```python
from build123d import *

# Parameters (mm, degrees)
EXTRUDE_1_DEPTH        = 110
FILLET_1_R             = 0.2
SKETCH_2_R             = 5.5
CUT_EXTRUDE_1_DEPTH    = 8
SKETCH_3_R             = 3.5
CUT_EXTRUDE_2_DEPTH    = 124.081273962
HOLE_WIZARD_M4_1_D     = 3.3
HOLE_WIZARD_M4_1_DEPTH = 16.5
HOLE_WIZARD_M4_1_TIP   = 0.991420021


with BuildPart() as part:
    # 스케치1 → 보스-돌출1 (new body)
    with BuildSketch(Plane(origin=(0, 0, 0), x_dir=(1, 0, 0), z_dir=(0, 1, 0))):
        Polygon((0, -43), (0, 0), (45, 0), (45, -40), (3, -40), (3, -43), align=None)
    extrude(amount=EXTRUDE_1_DEPTH)

    # 필렛1
    fillet_1_edges = [part.edges().sort_by_distance(p)[0] for p in [
        (3, 55, 40),
    ]]
    fillet(fillet_1_edges, radius=FILLET_1_R)

    # 스케치2 → 컷-돌출1 (cut)
    with BuildSketch(Plane.XY.offset(40)):
        with Locations((12.5, 75)):
            Circle(SKETCH_2_R)
        with Locations((35.5, 75)):
            Circle(SKETCH_2_R)
        with Locations((12.5, 35)):
            Circle(SKETCH_2_R)
        with Locations((35.5, 35)):
            Circle(SKETCH_2_R)
    extrude(amount=-CUT_EXTRUDE_1_DEPTH, mode=Mode.SUBTRACT)

    # 스케치3 → 컷-돌출2 (cut, through all)
    with BuildSketch(Plane.XY.offset(32)):
        with Locations((12.5, 75)):
            Circle(SKETCH_3_R)
        with Locations((35.5, 75)):
            Circle(SKETCH_3_R)
        with Locations((35.5, 35)):
            Circle(SKETCH_3_R)
        with Locations((12.5, 35)):
            Circle(SKETCH_3_R)
    extrude(amount=-CUT_EXTRUDE_2_DEPTH, mode=Mode.SUBTRACT)

    # M4 나사 구멍1
    with Locations(Plane.XY.offset(40)):
        with Locations((12.5, 95), (12.5, 15), (12.5, 55), (35.5, 55), (35.5, 95), (35.5, 15)):
            Hole(HOLE_WIZARD_M4_1_D / 2, depth=HOLE_WIZARD_M4_1_DEPTH)
            with Locations((0, 0, -(HOLE_WIZARD_M4_1_DEPTH + HOLE_WIZARD_M4_1_TIP / 2))):  # 118° drill point
                Cone(0, HOLE_WIZARD_M4_1_D / 2, HOLE_WIZARD_M4_1_TIP, mode=Mode.SUBTRACT)


solid = part.part
```
Verification items for the finished model (mm, model axes). A direction names the side the tool comes from. Give positions to 0.01 mm unless a question says otherwise; leave off trailing zeros. Order: outer loops, then holes, each group sorted by start corner. A loop starts at its lowest first (then second) coordinate and runs counter-clockwise, first axis right, second up. Notation, with made-up numbers: M -9.75,75.25 L 1.25,75.25 A21 ccw 1.25,82.25 Z; hole C 78.5,60 d4. An arc over 180 degrees is marked long. Return JSON: item names as keys, results as strings. Group by question number.
1) Scan lines: line 1 (Y direction, x = 35.5, z = 35.5); line 2 (Y direction, x = 12.5, z = 31.25); line 3 (X direction, y = 55, z = 34). Record each from-to range of solid material in increasing order.
2) Access from +Z, -Z, +X, -X, +Y, -Y to the whole of each face (thin tool, end or side, straight path). Record for faces 1 (the face through (34.741, 71.583, 16.224)), 2 (the face through (35, 31, 32)), 3 (the face through (24, 54, 40)).
3) Section check D-D on z = 33.5. Give the number of separate pieces and of enclosed holes in the cut face, and give its area (3 significant figures).
4) Section check B-B on z = 21. Record the cut outline in (x, y), and give its area (3 significant figures).
5) Mould release check, pull along X, two halves, no side actions. Record for faces 4 (the face through (35.9, 93.4, 31.6)), 5 (the face through (0, 54, 22)), 6 (the face through (2, 54, 43)): pulls with the +X half, pulls with the -X half, needs draft (parallel to the pull), parting line crosses it, or undercut.
6) Go/stop test with flat-tipped pins: pin 1 Ø12 at (x, y) = (34.5, 37) entering from +Z; pin 2 Ø2.5 at (x, y) = (35.5, 15) entering from +Z; pin 3 Ø5.5 at (x, y) = (33.5, 74) entering from +Z. Record where each tip stops, or that it passes through.
7) Section check C-C on y = 50. Record the cut outline in (x, z), and give its area (3 significant figures).
8) Section check A-A on y = 35. Record the cut outline in (x, z).
Answer block:
{
 "1": {"line 1": "y = 0 to 13.35, 16.65 to 29.5, 40.5 to 53.35, 56.65 to 69.5, 80.5 to 93.35, 96.65 to 110", "line 2": "y = 0 to 13.35, 16.65 to 31.5, 38.5 to 53.35, 56.65 to 71.5, 78.5 to 93.35, 96.65 to 110", "line 3": "x = 0 to 10.85, 14.15 to 33.85, 37.15 to 45"},
 "2": {"face 1": "+Z, -Z", "face 2": "+Z", "face 3": "+Z, +X, +Y, -Y"},
 "3": {"separate pieces": "1", "enclosed holes": "10", "area": "4,520 mm^2"},
 "4": {"outline": "M 0,0 L 45,0 L 45,110 L 0,110 Z; hole C 12.5,35 d7; hole C 12.5,75 d7; hole C 35.5,35 d7; hole C 35.5,75 d7", "area": "4,800 mm^2"},
 "5": {"face 4": "undercut", "face 5": "pulls with the -X half", "face 6": "needs draft"},
 "6": {"pin 1": "stops at z = 40", "pin 2": "stops at z = 23.26", "pin 3": "stops at z = 32"},
 "7": {"outline": "M 0,0 L 45,0 L 45,40 L 3.2,40 A0.2 cw 3,40.2 L 3,43 L 0,43 Z", "area": "1,810 mm^2"},
 "8": {"outline": "M 0,0 L 9,0 L 9,32 L 7,32 L 7,40 L 3.2,40 A0.2 cw 3,40.2 L 3,43 L 0,43 Z; M 16,0 L 32,0 L 32,32 L 30,32 L 30,40 L 18,40 L 18,32 L 16,32 Z; M 39,0 L 45,0 L 45,40 L 41,40 L 41,32 L 39,32 Z"}
}
